Geometry: see drawing. Coordinates: mm, zero at the bounding-box minimum. A direction names the side the tool comes from. Give positions to 0.01 mm unless a question says otherwise; leave off trailing zeros. Loops run counter-clockwise (first coordinate to the right, second up) from the corner with the lowest first, then second, coordinate; pieces in that order, holes last. Notation, with made-up numbers: (60.5, 10.25) -> (112.5, 10.25) arc R32 cw to (112.5, 43.25) -> close; hole circle Ø7 at (27, 88.25). An arc over 180 degrees is marked (long way). Use CSV: the item, a comma, the result in double quotes.
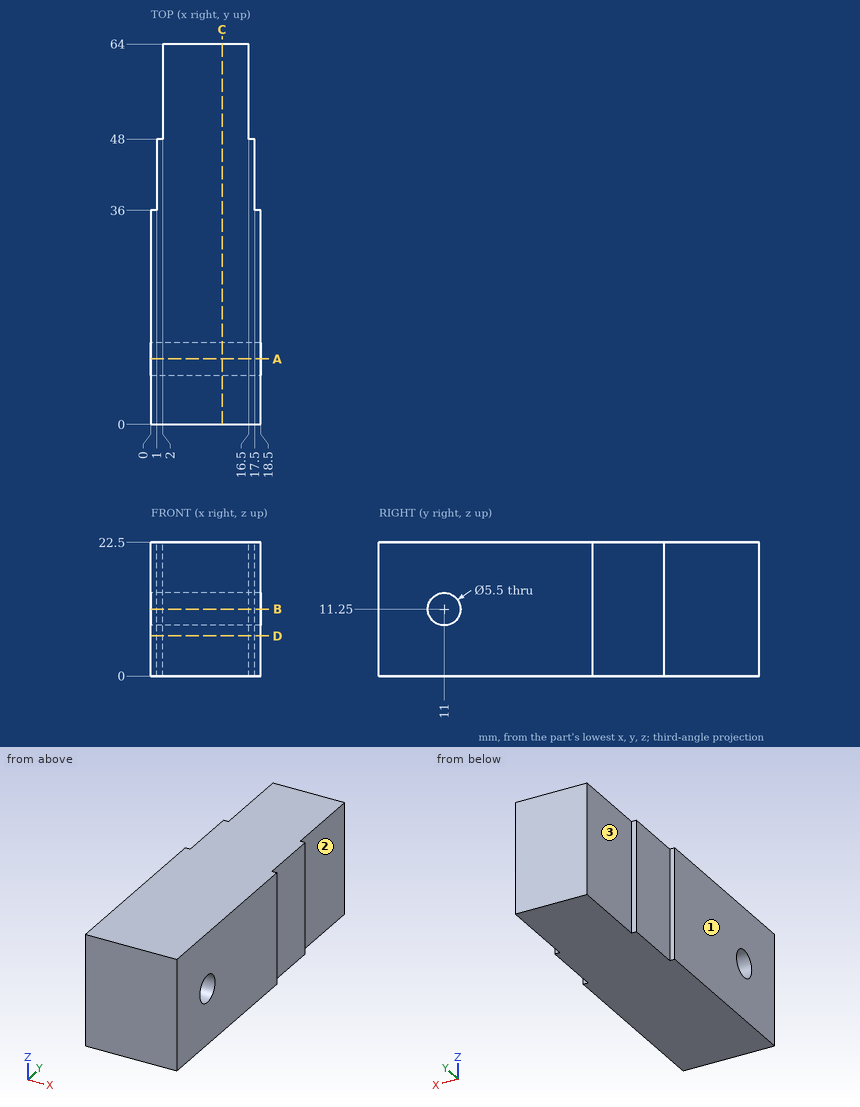
1) Contact query for flat-ended pins moving along their axis: pin 1 (1.1 mm diameter, centred on x = 18, z = 15, fed in from +Y); pin 2 (3.5 mm diameter, centred on y = 44, z = 9, fed in from +X); pin 3 (8 mm diameter, centred on y = 54.5, z = 15, fed in from -X). Output: stop coordinate, or through.
From the geometry:
pin 1,"stops at y = 48"
pin 2,"stops at x = 17.5"
pin 3,"stops at x = 2"
2) Section query A-A (y = 11). Return loops of the section in (x, z), then the cut area to 4 significant figures.
From the geometry:
outline,"(0, 0) -> (18.5, 0) -> (18.5, 8.5) -> (0, 8.5) -> close; (0, 14) -> (18.5, 14) -> (18.5, 22.5) -> (0, 22.5) -> close"
area,"314.5 mm^2"
3) Ray query, line 1 (X direction, y = 58, z = 18.75); line 2 (X direction, y = 40, z = 7.5); line 3 (Y direction, x = 11, z = 10). Return the intervals inside material, ascending.
From the geometry:
line 1,"x = 2 to 16.5"
line 2,"x = 1 to 17.5"
line 3,"y = 0 to 8.55, 13.45 to 64"
4) Section query C-C (x = 12). Return loops of the section in (y, z).
From the geometry:
outline,"(0, 0) -> (64, 0) -> (64, 22.5) -> (0, 22.5) -> close; hole circle Ø5.5 at (11, 11.25)"
5) Reachability of the marked faces 1, 2 and 3 from +Z, -Z, +X, -X, +Y, -Y: full face, straight path, thin tool, end or side. Return the list, or none.
From the geometry:
face 1,"+Z, -Z, -X, +Y, -Y"
face 2,"+Z, -Z, +X, +Y"
face 3,"+Z, -Z, -X, +Y"
6) Section query B-B (z = 11.25). Return loops of the section in (x, y).
From the geometry:
outline,"(0, 0) -> (18.5, 0) -> (18.5, 8.25) -> (0, 8.25) -> close; (0, 13.75) -> (18.5, 13.75) -> (18.5, 36) -> (17.5, 36) -> (17.5, 48) -> (16.5, 48) -> (16.5, 64) -> (2, 64) -> (2, 48) -> (1, 48) -> (1, 36) -> (0, 36) -> close"
7) Section query D-D (z = 6.75). Return loops of the section in (x, y), then the cut area to 3 significant figures.
From the geometry:
outline,"(0, 0) -> (18.5, 0) -> (18.5, 36) -> (17.5, 36) -> (17.5, 48) -> (16.5, 48) -> (16.5, 64) -> (2, 64) -> (2, 48) -> (1, 48) -> (1, 36) -> (0, 36) -> close"
area,"1,100 mm^2"
